from build123d import *

# Parameters (mm, degrees)
F0_R     = 9.525
F1_DEPTH = 87.9602
F2_W     = 159.8871313035
F2_H     = 188.4720697999
F2_W_2   = 68.9102
F2_H_2   = 63.5
F3_DEPTH = 101.601
F4_R     = 6.35
F5_DEPTH = 87.9612001
F6_DEPTH = 6.35


with BuildPart() as f1:
    # F0 (on Front) → F1 (new body)
    with BuildSketch(Plane.XZ):
        Polygon((50.8, 31.75), (-50.8, 31.75), (-50.8, 6.35), (-50.8, -31.75), (-9.525, -31.75), (0, -31.75), (9.525, -31.75), (50.8, -31.75), (50.8, 6.35), align=None)
        with BuildLine():
            ThreePointArc((9.525, -6.35), (6.7351920908, -13.0851920908), (0, -15.875))
            ThreePointArc((0, -15.875), (-6.7351920908, 0.3851920908), (9.525, -6.35))
        make_face(mode=Mode.SUBTRACT)
        with BuildLine():
            ThreePointArc((-15.875, 6.35), (-25.4, -3.175), (-34.925, 6.35))
            ThreePointArc((-34.925, 6.35), (-25.4, 15.875), (-15.875, 6.35))
        make_face(mode=Mode.SUBTRACT)
        with Locations((25.4, 6.35)):
            Circle(F0_R, mode=Mode.SUBTRACT)
        Polygon((0, -31.75), (-9.525, -31.75), (-9.525, -120.0502738357), (9.525, -119.6629032493), (9.525, -31.75), align=None)
        with BuildLine():
            ThreePointArc((9.525, -6.35), (-6.7351920908, 0.3851920908), (0, -15.875))
            ThreePointArc((0, -15.875), (6.7351920908, -13.0851920908), (9.525, -6.35))
        make_face()
    extrude(amount=F1_DEPTH)

    # F2 (on face) → F3 (cut, through all)
    with BuildSketch(Plane.YZ.offset(50.8)):
        with Locations((-38.3915323764, -28.8357771933)):
            Rectangle(F2_W, F2_H)
        with BuildLine():
            Line((-19.05, 31.75), (0, 31.75))
            Line((0, 31.75), (0, -31.75))
            Line((0, -31.75), (-11.43, -31.75))
            Line((-11.43, -31.75), (-11.43, -50.292))
            ThreePointArc((-11.43, -50.292), (-43.9381582579, -89.604562418), (-87.9602, -63.8302))
            Line((-87.9602, -63.8302), (-87.9602, -31.75))
            Line((-87.9602, -31.75), (-87.9602, 31.75))
            Line((-87.9602, 31.75), (-19.05, 31.75))
        make_face(mode=Mode.SUBTRACT)
        with Locations((-53.5051, 0)):
            Rectangle(F2_W_2, F2_H_2)
        with BuildLine():
            Line((-19.05, -50.292), (-19.05, -31.75))
            Line((-19.05, -31.75), (-87.9602, -31.75))
            Line((-87.9602, -31.75), (-87.9602, -63.8302))
            Line((-87.9602, -63.8302), (-80.3402, -63.8302))
            ThreePointArc((-80.3402, -63.8302), (-44.2580362559, -81.6757994644), (-19.05, -50.292))
        make_face()
    extrude(amount=-F3_DEPTH, mode=Mode.SUBTRACT)

    # F4
    f4_edges = [f1.edges().sort_by_distance(p)[0] for p in [
        (-50.8, -9.525, 31.75),
        (50.8, -9.525, 31.75),
        (50.8, -9.525, -31.75),
        (-50.8, -9.525, -31.75),
        (-9.525, -84.1502, -63.8302),
        (9.525, -84.1502, -63.8302),
    ]]
    fillet(f4_edges, radius=F4_R)

    # F0 (on Front) → F5 (cut, through all)
    with BuildSketch(Plane.XZ):
        with BuildLine():
            ThreePointArc((9.525, -6.35), (-6.7351920908, 0.3851920908), (0, -15.875))
            ThreePointArc((0, -15.875), (6.7351920908, -13.0851920908), (9.525, -6.35))
        make_face()
    extrude(amount=F5_DEPTH, mode=Mode.SUBTRACT)

    # F0 (on Front) → F6 (join)
    with BuildSketch(Plane.XZ):
        with BuildLine():
            ThreePointArc((9.525, -6.35), (-6.7351920908, 0.3851920908), (0, -15.875))
            ThreePointArc((0, -15.875), (6.7351920908, -13.0851920908), (9.525, -6.35))
        make_face()
    extrude(amount=F6_DEPTH)


solid = f1.part
Check sheet for the modelled part. Datum: model origin and axes. Units: mm. A direction names the side the tool comes from. Round coordinates to 2 decimals unless told otherwise and drop trailing zeros. Order: outer loops, then holes, each group sorted by start corner. A loop starts at its lowest first (then second) coordinate and runs counter-clockwise, first axis right, second up.
(1) Cross-section at B-B, the plane x = 25.4. Enter the section's corners in (y, z) (3 decimals), and give its area (3 significant figures).
(2) Go/stop test with flat-tipped pins: P1, Ø8, axis at x = 11, y = -18, coming from the -Z side; P2, Ø7, axis at x = 0, y = -83, coming from the +Z side; P3, Ø6, axis at x = 34, z = -21.5, coming from the -Y side. Record where each tip stops, or that it passes through.
(3) Cross-section at A-A, the plane z = 6.35. Enter the section's corners in (x, y) (3 decimals).
(4) Draft check along Y on faces 1 (the flat face through (1, -19.05, 8)), 2 (the flat face through (0, -84, -63.83)), 3 (the cylindrical face through (0.13, -44.85, -81.8)). Enter one of: pulls with the +Y half, pulls with the -Y half, needs draft (parallel to the pull), parting line crosses it, or undercut.
(5) Cross-section at D-D, the plane x = -32. Enter the section's corners in (y, z).
(6) Cross-section at C-C, the plane z = -6.35. Enter the section's corners in (x, y) (3 decimals), and give its area (3 significant figures).
(7) Scan lines: probe 1 along X at (y, z) = (-3, 6); probe 2 along X at (y, z) = (-9, -6); probe 3 along Z at (x, y) = (25, -7). Record each from-to range of solid material in increasing order.
(8) Access from +Z, -Z, +X, -X, +Y, -Y to the whole of each face (thin tool, end or side, straight path). Record for faces 4 (the flat face through (-9.525, -29, -74)), 5 (the flat face through (0, -11.43, -41)), 6 (the flat face through (0, -6.35, -6)), 7 (the flat face through (9.525, -34, -78)).
Check sheet entries:
1. outline: (-19.05, -31.75) - (0, -31.75) - (0, -3.175) - (-19.05, -3.175) - close; (-19.05, 15.875) - (0, 15.875) - (0, 31.75) - (-19.05, 31.75) - close
1. area: 847 mm2
2. P1: stops at z = -77.38
2. P2: stops at z = -63.83
2. P3: stops at y = -19.05
3. outline: (-50.8, -19.05) - (-34.925, -19.05) - (-34.925, 0) - (-50.8, 0) - close; (-15.875, -19.05) - (15.875, -19.05) - (15.875, 0) - (-15.875, 0) - close; (34.925, -19.05) - (50.8, -19.05) - (50.8, 0) - (34.925, 0) - close
4. face 1: pulls with the -Y half
4. face 2: needs draft
4. face 3: undercut
5. outline: (-19.05, -31.75) - (0, -31.75) - (0, -0.52) - (-19.05, -0.52) - close; (-19.05, 13.22) - (0, 13.22) - (0, 31.75) - (-19.05, 31.75) - close
6. outline: (-50.8, -19.05) - (-9.525, -19.05) - (-9.525, -6.35) - (9.525, -6.35) - (9.525, -19.05) - (50.8, -19.05) - (50.8, 0) - (-50.8, 0) - close
6. area: 1,690 mm2
7. probe 1: x = -50.8 to -34.92, -15.88 to 15.88, 34.92 to 50.8
7. probe 2: x = -50.8 to -9.52, 9.52 to 50.8
7. probe 3: z = -31.75 to -3.17, 15.87 to 31.75
8. face 4: -Z, -X, +Y, -Y
8. face 5: -Z, +X, -X, +Y
8. face 6: -Y
8. face 7: -Z, +X, +Y, -Y
